Autodesk Inventor part; units mm, degrees
ref_plane "YZ Plane" through (0, 0, 0) normal (1, 0, 0) x (0, 1, 0)
ref_plane "XZ Plane" through (0, 0, 0) normal (0, 1, 0) x (-1, 0, 0)
ref_plane "XY Plane" through (0, 0, 0) normal (0, 0, 1) x (1, 0, 0)
sketch "Sketch1" plane through (0, 0, 0) normal (1, 0, 0) x (0, 1, 0)
  circle A0 centre (0, 0) radius 14.2875
  circle A1 centre (0, -177.8) radius 14.2875
  line L0 (152.4, -31.75) -> (-152.4, -31.75) construction
  line L1 (-152.4, -31.75) -> (-152.4, -146.05) construction
  line L2 (-152.4, -146.05) -> (152.4, -146.05) construction
  line L3 (152.4, -146.05) -> (152.4, -31.75) construction
  line L4 (152.4, -31.75) -> (-152.4, -146.05) construction
  line L5 (-152.4, -31.75) -> (152.4, -146.05) construction
  circle A2 centre (0, 0) radius 38.1 construction
  circle A3 centre (0, -177.8) radius 38.1 construction
  circle A4 centre (0, 0) radius 31.75 construction
  circle A5 centre (0, -177.8) radius 31.75 construction
  circle A6 centre (0, 0) radius 26.9875 construction
  circle A7 centre (0, -177.8) radius 26.9875 construction
  circle A8 centre (97.4242, -177.8) radius 14.2875
  circle A9 centre (97.4242, -177.8) radius 38.1 construction
  circle A10 centre (97.4242, -177.8) radius 31.75 construction
  circle A11 centre (97.4242, -177.8) radius 26.9875 construction
  circle A12 centre (97.4242, 0) radius 14.2875
  circle A13 centre (97.4242, 0) radius 38.1 construction
  circle A14 centre (97.4242, 0) radius 31.75 construction
  circle A15 centre (97.4242, 0) radius 26.9875 construction
  line L6 (124.4117, -204.7875) -> (0, -204.7875)
  line L7 (124.4117, 26.9875) -> (0, 26.9875)
  line L8 (124.4117, 26.9875) -> (124.4117, -204.7875)
  line L9 (-26.9875, 0) -> (-26.9875, -177.8)
  arc A16 (0, 26.9875) -> (-26.9875, 0) centre (0, 0) ccw
  arc A17 (-26.9875, -177.8) -> (0, -204.7875) centre (0, -177.8) ccw
  line L10 (97.4242, -177.8) -> (0, -177.8) construction
  point P0 (0, -88.9)
  point P1 (97.4242, -204.7875)
  point P2 (124.4117, 0)
  point P3 (48.7121, 0)
  point P4 (48.7121, -177.8)
  point P5 (48.7121, -177.8)
  dimension "d0" = 28.575
  dimension "d2" = 304.8
  dimension "d3" = 114.3
  dimension "d4" = 76.2
  dimension "d6" = 6.35
  dimension "d7" = 12.7
  dimension "d8" = 97.4242
extrude "Extrusion1" add sketch "Sketch1" along normal blind 6.35
hole "Hole1" at (0, 48.7121, 0) at (0, 48.7121, -177.8) direction (1, 0, 0) diameter 5.1054 end through all
sketch "Sketch2" plane through (4.4901, 119.9216, 26.9875) normal (-0.7071068, 0.7071068, 0) x (-0.7071068, -0.7071068, 0)
  line L0 (0, -231.775) -> (0, 0)
  line L1 (0, 0) -> (-101.6, 0)
  line L2 (-101.6, 0) -> (-101.6, -231.775)
  line L3 (-101.6, -231.775) -> (0, -231.775)
edge flange "Flange1" height 101.6 angle 45 thickness 6.35 bend radius 6.35 thickness toward (-0.7071068, 0.7071068, 0) relief tear relief width 6.35 relief depth 3.175 edges at (6.35, 124.4117, -88.9) wall of the first edge with corners at (4.4901, 119.9216, -204.7875) (4.4901, 119.9216, 26.9875) (76.3322, 191.7637, 26.9875) (76.3322, 191.7637, -204.7875)
bend "Bend1"
corner "Corner1"
sketch "Sketch4" plane through (6.35, 0, 0) normal (1, 0, 0) x (0, 0, -1)
  circle A0 centre (0, 0) radius 14.2875 construction
  circle A1 centre (0, 0) radius 25.4 construction
  point P0 (0, 25.4)
  point P1 (-21.997, 12.7)
  point P2 (-21.997, -12.7)
  point P3 (0, -25.4)
  point P4 (21.997, -12.7)
  point P5 (21.997, 12.7)
  dimension "d38" = 50.8
  dimension "d41" = 360
hole "Hole3" at (6.35, 25.4, 0) at (6.35, 12.7, 21.997) at (6.35, -12.7, 21.997) at (6.35, -25.4, 0) at (6.35, -12.7, -21.997) at (6.35, 12.7, -21.997) direction (-1, 0, 0) diameter 5.1054 end through all
equation "\"d48\" = Thickness"
equation "\"d18\" = Thickness"
equation "\"d19\" = BendReliefWidth"
equation "\"d20\" = BendReliefDepth"
equation "\"d21\" = MinimumRemnant"
equation "\"d22\" = TransitionRadius"
equation "\"d25\" = BendRadius"
equation "\"d26\" = CornerReliefSize"
equation "\"d27\" = GapSize"
equation "\"d28\" = JacobiRadiusSize"
equation "\"BendRadius\" = Thickness"
equation "\"BendReliefWidth\" = Thickness"
equation "\"BendReliefDepth\" = 0.5 * Thickness"
equation "\"CornerReliefSize\" = 4 * Thickness"
equation "\"MinimumRemnant\" = 2 * Thickness"
equation "\"TransitionRadius\" = BendRadius"
equation "\"JacobiRadiusSize\" = BendRadius"
equation "\"GapSize\" = Thickness"
properties part number "GP4-005" material "Polycarbonate, Smoke"
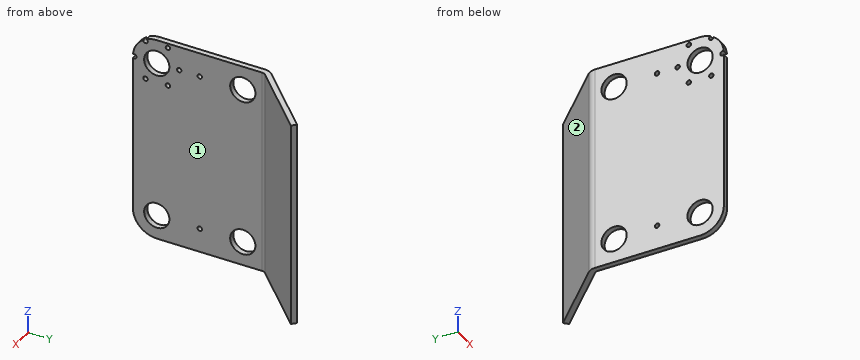
Check sheet for the modelled part. Datum: model origin and axes. Units: mm. Face numbers are marked on the shaded views. A direction names the side the tool comes from. Round coordinates to 2 decimals unless told otherwise and drop trailing zeros. Order: outer loops, then holes, each group sorted by start corner. A loop starts at its lowest first (then second) coordinate and runs counter-clockwise, first axis right, second up.
(1) Access from +Z, -Z, +X, -X, +Y, -Y to the whole of each face (thin tool, end or side, straight path). Record for the marked faces 1 and 2.
(2) Cross-section at C-C, the plane y = 61. Enter the section's corners in (x, z), and give its area (3 significant figures).
(3) Cross-section at A-A, the plane y = 6. Enter the section's corners in (x, z), and give its area (3 significant figures).
(4) Cross-section at B-B, the plane z = -105.5. Enter the section's corners in (x, y).
(5) Cross-section at D-D, the plane x = 17. Enter the section's corners in (y, z), and give its area (3 significant figures).
(6) Go/stop test with flat-tipped pins: P1, Ø3, axis at x = 29.5, z = -1.5, coming from the -Y side; P2, Ø4, axis at y = -25.4, z = 0, coming from the +X side; P3, Ø6.5, axis at y = 25.4, z = 0, coming from the +X side; P4, Ø6, axis at x = 45.5, z = -49.5, coming from the -Y side. Record where each tip stops, or that it passes through.
(7) Scan lines: probe 1 along Z at (x, y) = (3.25, 0); probe 2 along X at (y, z) = (7, -118.5); probe 3 along Y at (x, z) = (49, -169). Record each from-to range of solid material in increasing order.
Check sheet entries:
1. face 1: +Z, -Z, +X, -Y
1. face 2: +Z, -Z, -X, +Y
2. outline: (0, -204.79) - (6.35, -204.79) - (6.35, 26.99) - (0, 26.99) - close
2. area: 1,470 mm2
3. outline: (0, -204.79) - (6.35, -204.79) - (6.35, -190.77) - (0, -190.77) - close; (0, -164.83) - (6.35, -164.83) - (6.35, -12.97) - (0, -12.97) - close; (0, 12.97) - (6.35, 12.97) - (6.35, 26.99) - (0, 26.99) - close
3. area: 1,140 mm2
4. outline: (0, -26.99) - (6.35, -26.99) - (6.35, 119.15) arc R6.35 cw to (8.21, 123.64) - (76.33, 191.76) - (71.84, 196.25) - (3.72, 128.13) arc R12.7 ccw to (0, 119.15) - close
5. outline: (132.43, -204.79) - (141.41, -204.79) - (141.41, 26.99) - (132.43, 26.99) - close
5. area: 2,080 mm2
6. P1: stops at y = 143.43
6. P2: passes through
6. P3: stops at x = 6.35
6. P4: stops at y = 157.93
7. probe 1: z = -204.79 to -192.09, -163.51 to -14.29, 14.29 to 26.99
7. probe 2: x = 0 to 6.35
7. probe 3: y = 164.43 to 173.41
